Drawing for the job (mm, zero at the part's lowest x, y, z). A direction names the side the tool comes from. Coordinates: 2 decimals unless noted, no trailing zeros. Write each loop counter-clockwise with the first axis right and the second up, starting at its lowest first coordinate (ties: lowest second). Pieces come first, ordered by that corner, then holes. Notation, with made-up numbers: (11, -5.75) -> (16, -5.75) arc R19 ccw to (16, 22.25) -> close; hole circle Ø4 at (-35.75, 43). An arc over 180 degrees is marked (long way). Answer as CSV lines item,"result". Start each with the question number.
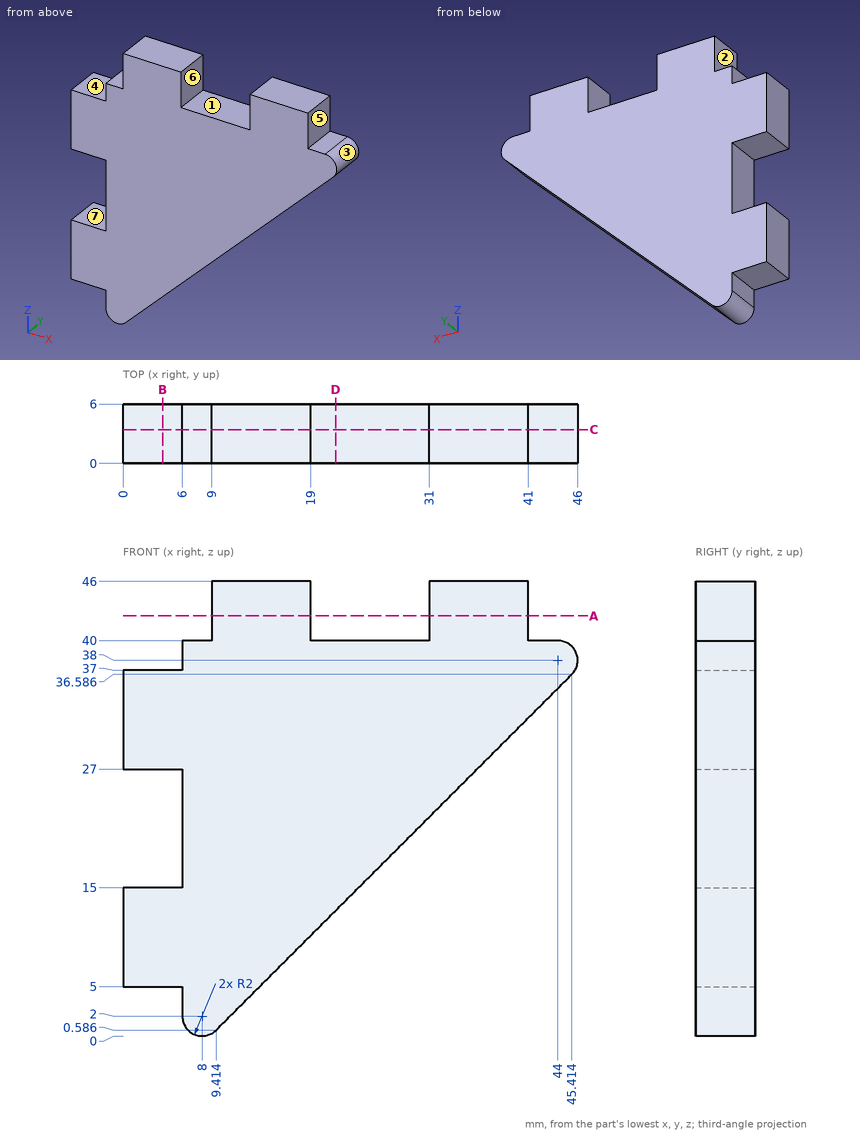
1. Wall check: line 1 (Z direction, x = 3, y = 1.3); line 2 (X direction, y = 4.2, z = 2.5); line 3 (X direction, y = 5.65, z = 11). Give the ranges that are in metal, low to high.
2. Flat gauge pins, fed straight in: P1, Ø2, axis at y = 4.5, z = 28.5, coming from the +X side; P2, Ø1.8, axis at y = 2.5, z = 23, coming from the -X side; P3, Ø1, axis at x = 18.5, y = 5, coming from the -Z side. Where does each tip first touch, or does it go through?
3. Cut at B-B (x = 4). Give the cut face in (y, z).
4. Cut at A-A (z = 42.5). Give the cut face in (x, y), then the cut area to 3 significant figures.
5. Cut at D-D (x = 21.5). Give the cut face in (y, z), then the cut area to 3 significant figures.
6. Mould opens along X. For the marked faces 1, 2, 3 and 4 say: pulls with the +X half, pulls with the -X half, needs draft (parallel to the pull), parting line crosses it, or undercut.
7. Cut at C-C (y = 3.4). Give the cut face in (x, z), then the cut area to 3 significant figures.
8. Tool access for the marked faces 5, 6 and 7: list every direction of +Z, -Z, +X, -X, +Y, -Y with a clear straight run to the whole face (end or side of a thin tool).
Geometry check:
1,line 1,"5 to 15, 27 to 37"
1,line 2,"6 to 11.33"
1,line 3,"0 to 19.83"
2,P1,"x = 38.33"
2,P2,"x = 6"
2,P3,"z = 9.17"
3,outline,"(0, 5) -> (6, 5) -> (6, 15) -> (0, 15) -> close; (0, 27) -> (6, 27) -> (6, 37) -> (0, 37) -> close"
4,outline,"(9, 0) -> (19, 0) -> (19, 6) -> (9, 6) -> close; (31, 0) -> (41, 0) -> (41, 6) -> (31, 6) -> close"
4,area,"120 mm²"
5,outline,"(0, 12.67) -> (6, 12.67) -> (6, 40) -> (0, 40) -> close"
5,area,"164 mm²"
6,face 1,"undercut"
6,face 2,"pulls with the -X half"
6,face 3,"pulls with the +X half"
6,face 4,"needs draft"
7,outline,"(0, 5) -> (6, 5) -> (6, 2) arc R2 ccw to (9.41, 0.59) -> (45.41, 36.59) arc R2 ccw to (44, 40) -> (41, 40) -> (41, 46) -> (31, 46) -> (31, 40) -> (19, 40) -> (19, 46) -> (9, 46) -> (9, 40) -> (6, 40) -> (6, 37) -> (0, 37) -> (0, 27) -> (6, 27) -> (6, 15) -> (0, 15) -> close"
7,area,"1,150 mm²"
8,face 5,"+Z, +X, +Y, -Y"
8,face 6,"+Z, +Y, -Y"
8,face 7,"-X, +Y, -Y"
